```python
from build123d import *

# Parameters (mm, degrees)
F0_W     = 330.2
F0_H     = 12.7
F0_R     = 2.032
F1_DEPTH = 12.7
F2_W     = 7.62
F2_H     = 7.62
F3_DEPTH = 424.18


with BuildPart() as f1:
    # F0 (on Top) → F1 (new body)
    with BuildSketch(Plane.XY):
        Rectangle(F0_W, F0_H)
        with Locations((-158.75, 0)):
            Circle(F0_R, mode=Mode.SUBTRACT)
        Circle(F0_R, mode=Mode.SUBTRACT)
        with Locations((158.75, 0)):
            Circle(F0_R, mode=Mode.SUBTRACT)
    extrude(amount=F1_DEPTH)

    # F2 (on face) → F3 (cut)
    with BuildSketch(Plane(origin=(-165.1, 0, 0), x_dir=(0, -1, 0), z_dir=(-1, 0, 0))):
        with Locations((0, 6.35)):
            Rectangle(F2_W, F2_H)
    extrude(amount=-F3_DEPTH, mode=Mode.SUBTRACT)


solid = f1.part
```
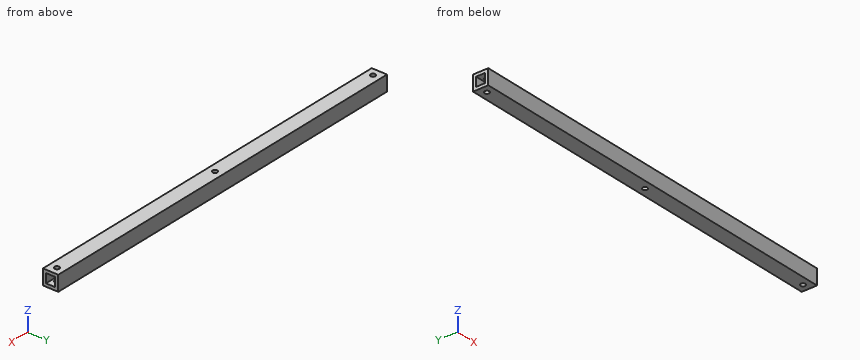
Model file for the job. Use its own axes, mm. Coordinates: 2 decimals unless noted, no trailing zeros. Loops run counter-clockwise (first coordinate to the right, second up) from the corner with the lowest first, then second, coordinate; pieces in that order, holes last. Notation, with made-up numbers: M 36,58.25 L 94,58.25 A28 cw 94,94.25 Z; hole C 82.25,-26 d6. An arc over 180 degrees is marked long. Use CSV: the item, a comma, the result in double quotes. Start each with the question number.
1. Band-saw the part on A-A, the plane z = 4.5. List the corners of the cut face in (x, y), then the cut area to 3 significant figures.
2. Probe probe 1 along X at (y, z) = (0, 11.15); probe 2 along Z at (x, y) = (96, 0.25); probe 3 along Y at (x, z) = (158.75, 11.15). List the from-to ranges inside material, lowest first. Write a range as [from, to].
3. Band-saw the part on B-B, the plane x = 79.5. List the corners of the cut face in (y, z).
Entries:
1,outline,"M -165.1,-6.35 L 165.1,-6.35 L 165.1,-3.81 L -165.1,-3.81 Z; M -165.1,3.81 L 165.1,3.81 L 165.1,6.35 L -165.1,6.35 Z"
1,area,"1,680 mm2"
2,probe 1,"x = [-165.1, -160.78], [-156.72, -2.03], [2.03, 156.72], [160.78, 165.1]"
2,probe 2,"z = [0, 2.54], [10.16, 12.7]"
2,probe 3,"y = [-6.35, -2.03], [2.03, 6.35]"
3,outline,"M -6.35,0 L 6.35,0 L 6.35,12.7 L -6.35,12.7 Z; hole M -3.81,2.54 L 3.81,2.54 L 3.81,10.16 L -3.81,10.16 Z"
